from build123d import *

# Parameters (mm, degrees)
SKETCH_W = 1
SKETCH_H = 5


with BuildPart() as part:
    # AdditivePipe: sweep along a path in Sketch001
    with BuildLine(Plane.XY) as additivepipe_path:
        Line((0, 0), (10, 0))
        ThreePointArc((10, 0), (13.535525, 1.464457), (15, 4.999975))
        Line((15, 4.999975), (15, 30.000013))
        ThreePointArc((15, 30.000013), (17.500007, 32.5), (20, 29.999999))
        Line((20, 29.999999), (20, 5.000002))
        ThreePointArc((20, 5.000002), (21.464465, 1.464467), (25, 0))
        Line((25, 0), (35, 0))
    # Sketch → AdditivePipe (sweep)
    with BuildSketch(Plane.YZ):
        with Locations((0, 2.5)):
            Rectangle(SKETCH_W, SKETCH_H)
    sweep(path=additivepipe_path.line)


solid = part.part
Check sheet for the modelled part. Datum: model origin and axes. Units: mm. A direction names the side the tool comes from. Round coordinates to 2 decimals unless told otherwise and drop trailing zeros. Loops run counter-clockwise (first coordinate to the right, second up) from the corner with the lowest first, then second, coordinate; pieces in that order, holes last. Notation, with made-up numbers: M 43.25,75 L 76.25,75 A12 ccw 76.25,93 Z; hole C -15,11 d4. An arc over 180 degrees is marked long. One line per question, with ' | ' between items. Start each with the question number.
Item 1: Scan lines: probe 1 along X at (y, z) = (10, 4.35); probe 2 along Y at (x, z) = (2, 1.9); probe 3 along X at (y, z) = (30.5, 4.2). Record each from-to range of solid material in increasing order.
Item 2: Section check B-B (z = 1.7). Record the boundary of the cut face in (x, y).
Item 3: Release check for a two-part mould opening along X. For faces 4 (the face through (19.5, 17, 3)), 5 (the face through (13.147, 1.783, 2.535)), 6 (the face through (35, 0, 3)) record: released by +X, released by -X, zero draft, split by the parting line, or undercut.
Item 4: Section check C-C (x = 17.5). Record the boundary of the cut face in (y, z), and give its area (3 significant figures).
Item 5: Set-up check for faces 1 (the face through (30, 0.5, 2)), 2 (the face through (21.07, 1.15, 2.47)), 3 (the face through (5, 0.5, 2)): record each of +Z, -Z, +X, -X, +Y, -Y from which the full face is reachable in a straight line by a thin tool's end or side.
Item 6: Section check A-A (y = 18.5). Record the boundary of the cut face in (x, z).
Item 7: Gauge pin test, flat ends, axial feed: pin 1 Ø3 at (y, z) = (12.5, 1) entering from +X; pin 2 Ø1.5 at (y, z) = (14.5, 2) entering from -X; pin 3 Ø2.5 at (x, z) = (30.5, 2.5) entering from +Y. Record the tip position at first contact, or that the pin passes through.
Worked out:
1) probe 1: 14.5 to 15.5, 19.5 to 20.5 | probe 2: -0.5 to 0.5 | probe 3: 14.54 to 15.56, 19.44 to 20.46
2) outline: M 0,-0.5 L 10,-0.5 A5.5 ccw 15.5,5 L 15.5,30 A2 cw 19.5,30 L 19.5,5 A5.5 ccw 25,-0.5 L 35,-0.5 L 35,0.5 L 25,0.5 A4.5 cw 20.5,5 L 20.5,30 A3 ccw 14.5,30 L 14.5,5 A4.5 cw 10,0.5 L 0,0.5 Z
3) face 4: undercut | face 5: released by -X | face 6: released by +X
4) outline: M 32,0 L 33,0 L 33,5 L 32,5 Z | area: 5.00 mm^2
5) face 1: +Z, -Z, +X, +Y | face 2: +Z, -Z, -Y | face 3: +Z, -Z, -X, +Y
6) outline: M 14.5,0 L 15.5,0 L 15.5,5 L 14.5,5 Z; M 19.5,0 L 20.5,0 L 20.5,5 L 19.5,5 Z
7) pin 1: x = 20.5 | pin 2: x = 14.5 | pin 3: y = 0.5
